CAD build for the part. Positions are in the model's coordinates, mm. Coordinates: 2 decimals unless noted, no trailing zeros. Write each loop counter-clockwise with the first axis right and the second up, starting at its lowest first coordinate (ties: lowest second). Pieces come first, ordered by that corner, then holes. Notation, with made-up numbers: (-8, -36) - (26, -36) arc R13 ccw to (26, -11) - close; hole circle Ø11 at (-32.75, 47). An arc over 180 degrees is marked (long way). One line per question, with ' | ' between items. Start each with the question number.
1. Band-saw the part on A-A, the plane y = 0. Write the cut outline in (x, z).
2. Flat gauge pins, fed straight in: P1, Ø2.5, axis at y = -77.95, z = 3, coming from the -X side; P2, Ø3, axis at x = 30.05, y = 30.05, coming from the +Z side; P3, Ø3.5, axis at y = 50.05, z = 3, coming from the +X side; P4, Ø1.5, axis at x = 6.5, z = 3.5, coming from the +Y side. Where does each tip first touch, or does it go through?
3. Band-saw the part on C-C, the plane y = 36.5. Write the cut outline in (x, z).
4. Probe line 1 (X direction, y = 51.5, z = 2.9); line 2 (Y direction, x = 58, z = 2.3); line 3 (Y direction, x = 0, z = 3). List the from-to ranges inside material, lowest first.
5. Band-saw the part on D-D, the plane z = 3. Give the number of separate pieces and of enclosed holes in the cut face, then the cut area to 3 significant figures.
6. Band-saw the part on B-B, the plane x = 0. Write the cut outline in (y, z).
from build123d import *

# Parameters (mm, degrees)
SKETCH_1_W          = 138
SKETCH_1_H          = 180
SKETCH_1_R          = 1.75
SKETCH_1_R_2        = 35
EXTRUDE_1_DEPTH     = 6
SKETCH_2_W          = 50
SKETCH_2_H          = 50
CUT_EXTRUDE_1_DEPTH = 10
SKETCH_4_W          = 185.340515344
SKETCH_4_H          = 73.1161564
CUT_EXTRUDE_3_DEPTH = 10
SKETCH_3_R          = 1.5
CUT_EXTRUDE_2_DEPTH = 15


with BuildPart() as part:
    # 草图1 → 凸台-拉伸1 (new body)
    with BuildSketch(Plane.XY):
        Rectangle(SKETCH_1_W, SKETCH_1_H)
        with Locations((0, 42.5)):
            Circle(SKETCH_1_R, mode=Mode.SUBTRACT)
        with Locations((30.0520382, 30.0520382)):
            Circle(SKETCH_1_R, mode=Mode.SUBTRACT)
        with Locations((42.5, 0)):
            Circle(SKETCH_1_R, mode=Mode.SUBTRACT)
        with Locations((30.0520382, -30.0520382)):
            Circle(SKETCH_1_R, mode=Mode.SUBTRACT)
        with Locations((0, -42.5)):
            Circle(SKETCH_1_R, mode=Mode.SUBTRACT)
        with Locations((-30.0520382, -30.0520382)):
            Circle(SKETCH_1_R, mode=Mode.SUBTRACT)
        with Locations((-42.5, 0)):
            Circle(SKETCH_1_R, mode=Mode.SUBTRACT)
        with Locations((-30.0520382, 30.0520382)):
            Circle(SKETCH_1_R, mode=Mode.SUBTRACT)
        Circle(SKETCH_1_R_2, mode=Mode.SUBTRACT)
    extrude(amount=EXTRUDE_1_DEPTH)

    # 草图2 → 切除-拉伸1 (cut)
    with BuildSketch(Plane(origin=(0, 0, 0), x_dir=(-1, 0, 0), z_dir=(0, 0, -1))):
        with Locations((0, 45)):
            Rectangle(SKETCH_2_W, SKETCH_2_H)
    extrude(amount=-CUT_EXTRUDE_1_DEPTH, mode=Mode.SUBTRACT)

    # 草图4 → 切除-拉伸3 (cut)
    with BuildSketch(Plane(origin=(0, 0, 0), x_dir=(-1, 0, 0), z_dir=(0, 0, -1))):
        with Locations((5.331713455, 101.6101164)):
            Rectangle(SKETCH_4_W, SKETCH_4_H)
    extrude(amount=-CUT_EXTRUDE_3_DEPTH, mode=Mode.SUBTRACT)

    # 草图3 → 切除-拉伸2 (cut)
    with BuildSketch(Plane.ZY.offset(69)):
        with Locations(Location((3, 50.0520382, 0), (0, 0, 270))):
            Circle(SKETCH_3_R)
        with Locations(Location((3, 18.0520382, 0), (0, 0, 270))):
            Circle(SKETCH_3_R)
        with Locations(Location((3, -13.9479618, 0), (0, 0, 270))):
            Circle(SKETCH_3_R)
        with Locations(Location((3, -45.9479618, 0), (0, 0, 270))):
            Circle(SKETCH_3_R)
        with Locations(Location((3, -77.9479618, 0), (0, 0, 270))):
            Circle(SKETCH_3_R)
    cut_extrude_2 = extrude(amount=-CUT_EXTRUDE_2_DEPTH, mode=Mode.SUBTRACT)

    # 镜向1: 切除-拉伸2 across plane
    add(cut_extrude_2.mirror(Plane.ZY), mode=Mode.SUBTRACT)


solid = part.part
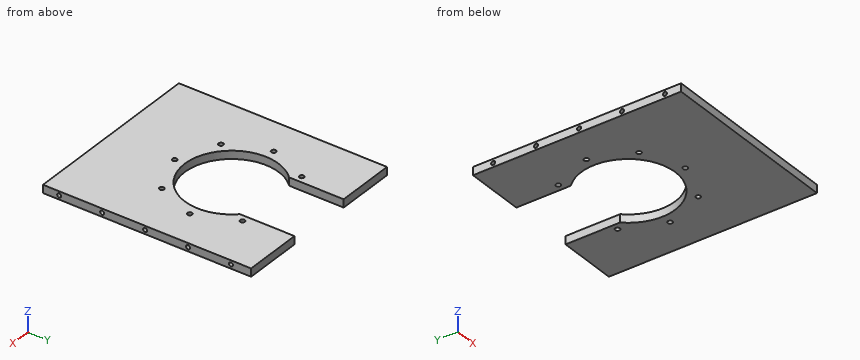
Filled in:
1) outline: (-69, 0) - (-44.25, 0) - (-44.25, 6) - (-69, 6) - close; (-40.75, 0) - (-35, 0) - (-35, 6) - (-40.75, 6) - close; (35, 0) - (40.75, 0) - (40.75, 6) - (35, 6) - close; (44.25, 0) - (69, 0) - (69, 6) - (44.25, 6) - close
2) P1: stops at x = -54 | P2: passes through | P3: stops at x = 69 | P4: stops at y = -34.24
3) outline: (-69, 0) - (-25, 0) - (-25, 6) - (-69, 6) - close; (25, 0) - (69, 0) - (69, 6) - (25, 6) - close
4) line 1: x = -54 to -25, 25 to 54 | line 2: y = -90 to -79.27, -76.62 to -47.27, -44.62 to -15.27, -12.62 to 16.73, 19.38 to 48.73, 51.38 to 65.05 | line 3: y = -90 to -44.25, -40.75 to -35
5) separate pieces: 1 | enclosed holes: 7 | area: 15,400 mm²
6) outline: (-90, 0) - (-44.25, 0) - (-44.25, 6) - (-90, 6) - close; (-40.75, 0) - (-35, 0) - (-35, 6) - (-40.75, 6) - close
